Work out the finished part from the listing and answer in its coordinate system (mm). Face numbers are marked on the shaded views. A direction names the side the tool comes from. Give positions to 0.01 mm unless a question says otherwise; leave off trailing zeros. Loops run counter-clockwise (first coordinate to the right, second up) from the corner with the lowest first, then second, coordinate; pieces in that order, holes last. Notation, with made-up numbers: M 34,88.25 L 81,88.25 A17 ccw 81,104.25 Z; hole C -18.75,82 d9. An arc over 180 degrees is marked long. Use a Markdown table: item, result.
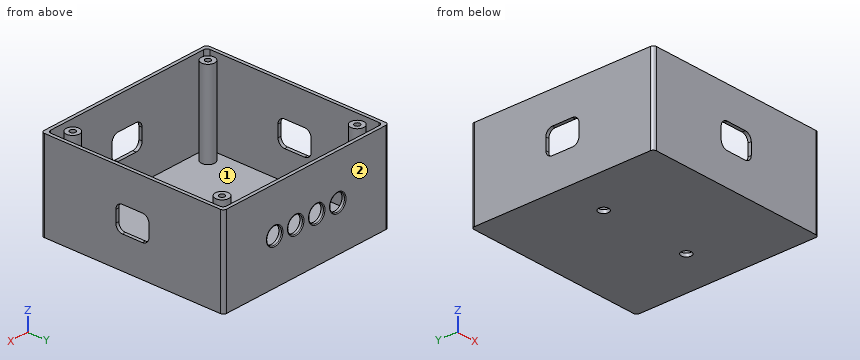
Autodesk Inventor part; units mm, degrees
ref_plane "YZ Plane" through (0, 0, 0) normal (1, 0, 0) x (0, 1, 0)
ref_plane "XZ Plane" through (0, 0, 0) normal (0, 1, 0) x (-1, 0, 0)
ref_plane "XY Plane" through (0, 0, 0) normal (0, 0, 1) x (1, 0, 0)
sketch "Sketch1" plane through (0, 0, 0) normal (0, 0, 1) x (1, 0, 0)
  line L0 (-55, -55) -> (55, -55)
  line L1 (55, -55) -> (55, 55)
  line L2 (55, 55) -> (-55, 55)
  line L3 (-55, 55) -> (-55, -55)
  line L4 (-55, -55) -> (55, 55) construction
  line L5 (55, -55) -> (-55, 55) construction
  point P0 (0, 0)
  dimension "Base_Width" = 110
  dimension "Base_Length" = 110
extrude "BaseBottom" add sketch "Sketch1" along normal blind 2
sketch "Sketch9" plane through (0, 0, 2) normal (0, 0, 1) x (1, 0, 0)
  line L0 (55, 55) -> (-55, 55)
  line L1 (0, 55) -> (0, -55) construction
  line L2 (-55, -55) -> (55, -55)
  circle A0 centre (-27.5, 0) radius 3
  circle A1 centre (27.5, 0) radius 3
  point P0 (0, 0)
  point P1 (0, 0)
  dimension "WallMount_Hole_Diameter" = 6
  dimension "WallMount_Hole_XPosition" = 27.5
  dimension "WallMount_Hole_YPosition" = 0
extrude "WallMountHoles" cut sketch "Sketch9" against normal up to surface (2 mm away)
sketch "Sketch3" plane through (0, 0, 2) normal (0, 0, 1) x (1, 0, 0)
  line L0 (55, -55) -> (55, 55)
  line L1 (-55, -55) -> (55, -55)
  line L2 (55, -55) -> (55, 55)
  line L3 (55, 55) -> (-55, 55)
  line L4 (-55, 55) -> (-55, -55)
  line L5 (-55, -55) -> (55, 55) construction
  line L6 (55, -55) -> (-55, 55) construction
  line L7 (-53, 53) -> (53, 53)
  line L8 (53, 53) -> (53, -53)
  line L9 (53, -53) -> (-53, -53)
  line L10 (-53, -53) -> (-53, 53)
  point P0 (0, 0)
  dimension "Base_Wall_Thickness" = 2
extrude "BaseWalls" add sketch "Sketch3" along normal blind 51
sketch "Sketch4" plane through (-55, -55, 0) normal (0, -1, 0) x (1, 0, 0)
  line L0 (45, 19) -> (65, 19)
  line L1 (65, 19) -> (65, 34)
  line L2 (65, 34) -> (45, 34)
  line L3 (45, 34) -> (45, 19)
  line L4 (45, 19) -> (65, 34) construction
  line L5 (65, 19) -> (45, 34) construction
  line L6 (55, 0) -> (55, 53) construction
  line L7 (2, 53) -> (108, 53)
  point P0 (55, 26.5)
  dimension "BatteryConnector_Hole_Width" = 20
  dimension "BatteryConnector_Hole_Height" = 15
extrude "BatteryConnectorHole" cut sketch "Sketch4" against normal up to surface (2 mm away)
sketch "Sketch5" plane through (55, -55, 0) normal (1, 0, 0) x (0, 0, -1)
  line L0 (0, 55) -> (-53, 55) construction
  line L1 (-53, 2) -> (-53, 108)
  line L2 (-19, 45) -> (-34, 45)
  line L3 (-34, 45) -> (-34, 65)
  line L4 (-34, 65) -> (-19, 65)
  line L5 (-19, 65) -> (-19, 45)
  line L6 (-19, 45) -> (-34, 65) construction
  line L7 (-34, 45) -> (-19, 65) construction
  point P0 (-26.5, 55)
  dimension "GridConnector_Hole_Width" = 20
  dimension "GridConnector_Hole_Height" = 15
extrude "GridConnectorHole" cut sketch "Sketch5" against normal up to surface (2 mm away)
sketch "Sketch6" plane through (-55, -55, 0) normal (-1, 0, 0) x (0, 0, 1)
  line L0 (0, 55) -> (53, 55) construction
  line L1 (53, 2) -> (53, 108)
  line L2 (19, 65) -> (34, 65)
  line L3 (34, 65) -> (34, 45)
  line L4 (34, 45) -> (19, 45)
  line L5 (19, 45) -> (19, 65)
  line L6 (19, 65) -> (34, 45) construction
  line L7 (34, 65) -> (19, 45) construction
  point P0 (26.5, 55)
  dimension "DeviceConnector_Hole_Width" = 20
  dimension "DeviceConnector_Hole_Height" = 15
extrude "DeviceConnectorHole" cut sketch "Sketch6" against normal up to surface (2 mm away)
sketch "Sketch8" plane through (-55, 55, 0) normal (0, 1, 0) x (1, 0, 0)
  line L0 (0, 0) -> (0, -53)
  line L1 (0, -26.5) -> (110, -26.5) construction
  line L2 (110, 0) -> (110, -53)
  circle A0 centre (34, -26.5) radius 5
  circle A1 centre (48, -26.5) radius 5
  circle A2 centre (62, -26.5) radius 5
  circle A3 centre (76, -26.5) radius 5
  point P0 (55, 0)
  point P1 (55, -26.5)
  dimension "Distance_Between_Buttons" = 14
  dimension "Button_Hole_Diameter" = 10
  dimension "Center_Buttons" = 21
extrude "ButtonHoles" cut sketch "Sketch8" against normal up to surface (2 mm away)
fillet "BaseCorners" radius 2 8 edges at (-55, 55, 26.5) (55, 55, 26.5) (55, -55, 26.5) (-55, -55, 26.5) (-53, -53, 27.5) (-53, 53, 27.5) (53, 53, 27.5) (53, -53, 27.5)
sketch "Sketch11" plane through (0, 0, 2) normal (0, 0, 1) x (1, 0, 0)
  circle A0 centre (-45, 45) radius 4
  line L0 (53, 55) -> (-53, 55)
  line L1 (-55, 53) -> (-55, -53)
  line L2 (0, 0) -> (0, 55) construction
  line L3 (0, 0) -> (-55, 0) construction
  circle A1 centre (45, 45) radius 4
  circle A2 centre (-45, -45) radius 4
  circle A3 centre (45, -45) radius 4
  dimension "d64" = 8
  dimension "d65" = 10
  dimension "d66" = 10
extrude "Extrusion11" add sketch "Sketch11" along normal blind 51
sketch "Sketch12" plane through (-45, 45, 53) normal (0, 0, 1) x (1, 0, 0)
  circle A0 centre (90, -90) radius 4
  circle A1 centre (90, -90) radius 1.65
  circle A2 centre (0, 0) radius 1.65
  circle A3 centre (90, 0) radius 1.65
  circle A4 centre (0, -90) radius 1.65
  circle A5 centre (0, -90) radius 4
  circle A6 centre (0, 0) radius 4
  circle A7 centre (90, 0) radius 4
  point P0 (45, -45)
  dimension "d69" = 3.3
  dimension "d70" = 3.3
  dimension "d71" = 3.3
  dimension "d72" = 3.3
  dimension "d73" = 0
  dimension "d74" = 0
  dimension "d75" = 0
  dimension "d76" = 0
  dimension "d77" = 0
  dimension "d78" = 0
extrude "Extrusion12" cut sketch "Sketch12" against normal blind 20 contours A1 | A2 | A3 | A4
fillet "Fillet2" radius 0.5 4 edges at (16, 55, 26.5) (2, 55, 26.5) (-12, 55, 26.5) (-26, 55, 26.5)
fillet "Fillet3" radius 4 12 edges at (54, 10, 34) (54, 10, 19) (54, -10, 34) (54, -10, 19) (-10, -54, 19) (10, -54, 19) (-10, -54, 34) (10, -54, 34) (-54, 10, 19) (-54, 10, 34) (-54, -10, 19) (-54, -10, 34)
equation "\"Base_Width\" = PCB_Width + 2 * Offset"
equation "\"Base_Length\" = PCB_Length + 2 * Offset"
equation "\"Base_Bottom_Thickness\" = Wall_Thickness"
equation "\"Base_Wall_Thickness\" = Wall_Thickness"
equation "\"Base_Height\" = Offset + PCB_Height - 2 * Wall_Thickness"
equation "\"d15\" = PCB_Height + Offset"
equation "\"Distance_Between_Buttons\" = Button_Diameter + Button_Distance_Between"
equation "\"Button_Hole_Diameter\" = Button_Diameter"
equation "\"d37\" = Wall_Thickness"
equation "\"d67\" = Offset + PCB_Height - 2 * Wall_Thickness"
properties part number "Base"
(1) Given P1, Ø1.6, axis at x = -44.5, y = 45, coming from the +Z side; P2, Ø5, axis at x = -27.5, y = 0, coming from the -Z side; P3, Ø0.6, axis at x = -54.5, z = 28, coming from the -Y side; P4, Ø0.6, axis at y = -54, z = 26.5, coming from the +X side, each flat-ended and moving along its own axis, determine where each tip first touches the part or whether it passes through.
Entries:
| item | result |
|---|---|
| P1 | stops at z = 33 |
| P2 | passes through |
| P3 | stops at y = -54.6 |
| P4 | stops at x = 54.87 |
(2) Which of the six approach directions +Z, -Z, +X, -X, +Y, -Y give full straight-line access (tool end or side, diameter ignored) to the marked faces 1 and 2?
Entries:
| item | result |
|---|---|
| face 1 | +Z |
| face 2 | +Z, -Z, +X, -X, +Y |
(3) A cutting plane is placed at B-B (z = 48.5). Count the separate pieces of the cut face and the enclosed holes in it, and give its area (3 significant figures).
Entries:
| item | result |
|---|---|
| separate pieces | 5 |
| enclosed holes | 5 |
| area | 1,030 mm² |
(4) Consider probe 1 along Y at (x, z) = (45, 46); probe 2 along Y at (x, z) = (15, 45.5); probe 3 along Y at (x, z) = (-27.5, 0.55). Determine where each line is inside the solid, lowest interval first. Write a range as [from, to].
Entries:
| item | result |
|---|---|
| probe 1 | y = [-55, -53], [-49, -46.65], [-43.35, -41], [41, 43.35], [46.65, 49], [53, 55] |
| probe 2 | y = [-55, -53], [53, 55] |
| probe 3 | y = [-55, -3], [3, 55] |
(5) A cutting plane is placed at A-A (z = 10). Write down the section's boundary in (x, y).
Entries:
| item | result |
|---|---|
| outline | M -55,-53 A2 ccw -53,-55 L 53,-55 A2 ccw 55,-53 L 55,53 A2 ccw 53,55 L -53,55 A2 ccw -55,53 Z; C -45,-45 d8; C -45,45 d8; C 45,-45 d8; C 45,45 d8; hole M -53,-51 A2 ccw -51,-53 L 51,-53 A2 ccw 53,-51 L 53,51 A2 ccw 51,53 L -51,53 A2 ccw -53,51 Z |
(6) A cutting plane is placed at D-D (y = 18.5). Write down the section's boundary in (x, z), and give its area (3 significant figures).
Entries:
| item | result |
|---|---|
| outline | M -55,0 L 55,0 L 55,53 L 53,53 L 53,2 L -53,2 L -53,53 L -55,53 Z |
| area | 424 mm² |
(7) A cutting plane is placed at C-C (x = -45). Write down the section's boundary in (y, z), and give its area (3 significant figures).
Entries:
| item | result |
|---|---|
| outline | M -55,0 L 55,0 L 55,53 L 53,53 L 53,2 L 49,2 L 49,53 L 46.65,53 L 46.65,33 L 43.35,33 L 43.35,53 L 41,53 L 41,2 L -41,2 L -41,53 L -43.35,53 L -43.35,33 L -46.65,33 L -46.65,53 L -49,53 L -49,2 L -53,2 L -53,53 L -55,53 Z |
| area | 1,110 mm² |
